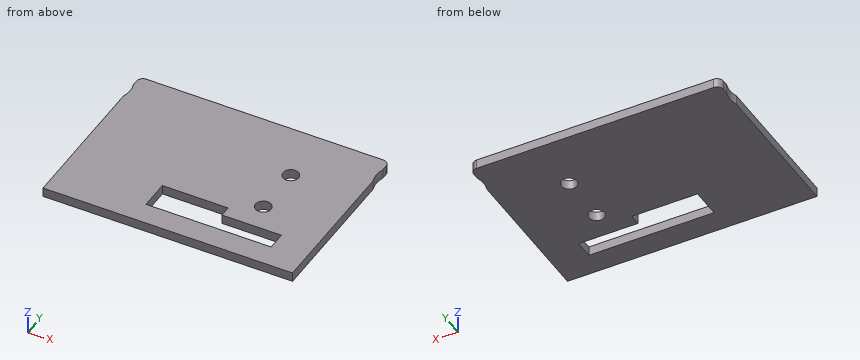
```python
from build123d import *

# Parameters (mm, degrees)
SKETCH2_W           = 80
SKETCH2_H           = 56.8
SKETCH2_R           = 2.5
BOSS_EXTRUDE1_DEPTH = 3
SKETCH4_W           = 0.125
SKETCH4_H           = 56.8
CUT_EXTRUDE2_DEPTH  = 99.159258351
SKETCH3_R           = 8.5
CUT_EXTRUDE1_DEPTH  = 99.057409842
FILLET1_R           = 2


with BuildPart() as part:
    # Sketch2 → Boss-Extrude1 (new body)
    with BuildSketch(Plane.XY):
        with Locations((40, 28.4)):
            Rectangle(SKETCH2_W, SKETCH2_H)
        with Locations((58.4, 38.35)):
            Circle(SKETCH2_R, mode=Mode.SUBTRACT)
        with Locations((58.4, 22.25)):
            Circle(SKETCH2_R, mode=Mode.SUBTRACT)
        Polygon((29, 7.4), (29, 17), (50, 17), (50, 13.4), (69, 13.4), (69, 7.4), align=None, mode=Mode.SUBTRACT)
    extrude(amount=BOSS_EXTRUDE1_DEPTH)

    # Sketch4 → Cut-Extrude2 (cut, through all)
    with BuildSketch(Plane.XY.offset(3)):
        with Locations((0.0625, 28.4)):
            Rectangle(SKETCH4_W, SKETCH4_H)
        with Locations((79.9375, 28.4)):
            Rectangle(SKETCH4_W, SKETCH4_H)
    extrude(amount=-CUT_EXTRUDE2_DEPTH, mode=Mode.SUBTRACT)

    # Sketch3 → Cut-Extrude1 (cut, through all)
    with BuildSketch(Plane.XY.offset(3)):
        with Locations((-7.875, 50)):
            Circle(SKETCH3_R)
        with Locations((87.875, 50)):
            Circle(SKETCH3_R)
    extrude(amount=-CUT_EXTRUDE1_DEPTH, mode=Mode.SUBTRACT)

    # Fillet1
    fillet1_edges = [part.edges().sort_by_distance(p)[0] for p in [
        (0.125, 56.8, 1.5),
        (79.875, 56.8, 1.5),
    ]]
    fillet(fillet1_edges, radius=FILLET1_R)


solid = part.part
```
The model under review builds one solid part; all positions refer to its coordinate system, in mm. Round coordinates to 2 decimals unless told otherwise and drop trailing zeros. Order: outer loops, then holes, each group sorted by start corner. A loop starts at its lowest first (then second) coordinate and runs counter-clockwise, first axis right, second up. Notation, with made-up numbers: (43.25, 85.5) - (62.25, 85.5) arc R9 ccw to (62.25, 94.5) - close; hole circle Ø2 at (85, -39). An arc over 180 degrees is marked (long way). Answer in a Markdown table with one row per item.
(1) Take a section at C-C on z = 2.1. Write out the cut boundary in (x, y) (3 decimals), plus the area to 3 significant figures.
Result set:
| item | result |
|---|---|
| outline | (0.125, 0) - (79.875, 0) - (79.875, 47.128) arc R8.5 cw to (79.875, 52.872) - (79.875, 54.8) arc R2 ccw to (77.875, 56.8) - (2.125, 56.8) arc R2 ccw to (0.125, 54.8) - (0.125, 52.872) arc R8.5 cw to (0.125, 47.128) - close; hole (29, 7.4) - (69, 7.4) - (69, 13.4) - (50, 13.4) - (50, 17) - (29, 17) - close; hole circle Ø5 at (58.4, 22.25); hole circle Ø5 at (58.4, 38.35) |
| area | 4,170 mm2 |
(2) Take a section at D-D on x = 42.5. Write out the cut boundary in (y, z), plus the area to 3 significant figures.
Result set:
| item | result |
|---|---|
| outline | (0, 0) - (7.4, 0) - (7.4, 3) - (0, 3) - close; (17, 0) - (56.8, 0) - (56.8, 3) - (17, 3) - close |
| area | 142 mm2 |
(3) Clearance check with a flat-ended pin moving along its axis: P1, Ø4, axis at x = 58.4, y = 22.25, coming from the +Z side. State where the tip first meets the part, or that it passes through.
Result set:
| item | result |
|---|---|
| P1 | passes through |
(4) For line 1 (Y direction, x = 58.4, z = 1.95); line 2 (X direction, y = 8, z = 0.4) (3 decimals); line 3 (X direction, y = 14, z = 0.4) (3 decimals), list the stretches that pass through material, from the lowest coordinate up. Write a range as from..to.
Result set:
| item | result |
|---|---|
| line 1 | y = 0..7.4, 13.4..19.75, 24.75..35.85, 40.85..56.8 |
| line 2 | x = 0.125..29, 69..79.875 |
| line 3 | x = 0.125..29, 50..79.875 |
(5) Take a section at B-B on y = 38.35. Write out the cut boundary in (x, z) (3 decimals), plus the area to 3 significant figures.
Result set:
| item | result |
|---|---|
| outline | (0.125, 0) - (55.9, 0) - (55.9, 3) - (0.125, 3) - close; (60.9, 0) - (79.875, 0) - (79.875, 3) - (60.9, 3) - close |
| area | 224 mm2 |
(6) Take a section at A-A on x = 58.4. Write out the cut boundary in (y, z), plus the area to 3 significant figures.
Result set:
| item | result |
|---|---|
| outline | (0, 0) - (7.4, 0) - (7.4, 3) - (0, 3) - close; (13.4, 0) - (19.75, 0) - (19.75, 3) - (13.4, 3) - close; (24.75, 0) - (35.85, 0) - (35.85, 3) - (24.75, 3) - close; (40.85, 0) - (56.8, 0) - (56.8, 3) - (40.85, 3) - close |
| area | 122 mm2 |
